Check sheet for the modelled part. Datum: model origin and axes. Units: mm. Face numbers are marked on the shaded views. A direction names the side the tool comes from. Round coordinates to 2 decimals unless told otherwise and drop trailing zeros. Write item = value, one per line.
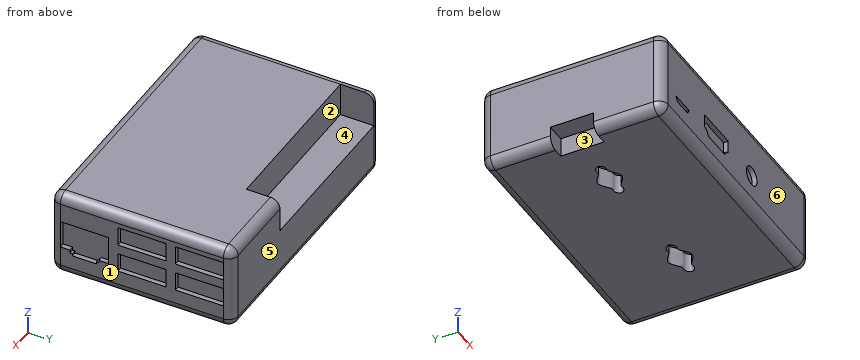
from build123d import *

# Parameters (mm, degrees)
F0_W     = 6.35
F0_H     = 7.14375
F1_DEPTH = 28.575
F2_DEPTH = 6.35
F4_W     = 15.875
F4_H     = 6.35
F5_DEPTH = 1.5875
F3_R     = 3.175
F6_DEPTH = 1.5875
F7_W     = 57.15
F7_H     = 11.1125
F8_DEPTH = 11.1125
F9_R     = 3.17499


# Not quite as in the source:
# - a fillet or chamfer is up to 0.001 mm smaller than in the source, because OpenCascade refuses the exact size


with BuildPart() as f1:
    # F0 (on Top) → F1 (new body)
    with BuildSketch(Plane.XY):
        Polygon((44.45, -30.1625), (44.45, 30.1625), (-44.45, 30.1625), (-44.45, 7.14375), (-38.1, 7.14375), (-38.1, 0), (-38.1, -7.14375), (-44.45, -7.14375), (-44.45, -30.1625), align=None)
        with BuildLine():
            add(Edge.make_bspline(
                [(-14.2875, 0), (-14.2875, 0.7324493897), (-15.9479784808, 2.0808128457), (-17.5976715514, 0.8021829538), (-21.43125, 5.9657530394), (-25.2648284486, 0.8021829538), (-26.9145215192, 2.0808128457), (-29.4769945213, 0), (-26.9145215192, -2.0808128457), (-25.2648284486, -0.8021829538), (-21.43125, -5.9657530394), (-17.5976715514, -0.8021829538), (-15.9479784808, -2.0808128457), (-14.2875, -0.7324493897), (-14.2875, 0)],
                knots=[0, 0, 0, 0, 0.0762961044, 0.1404532251, 0.25, 0.3595467749, 0.4237038956, 0.5, 0.5762961044, 0.6404532251, 0.75, 0.8595467749, 0.9237038956, 1, 1, 1, 1], degree=3))
        make_face(mode=Mode.SUBTRACT)
        with BuildLine():
            add(Edge.make_bspline(
                [(14.2875, 0), (14.2875, 0.7324493897), (15.9479784808, 2.0808128457), (17.5976715514, 0.8021829538), (21.43125, 5.9657530394), (25.2648284486, 0.8021829538), (26.9145215192, 2.0808128457), (29.4769945213, 0), (26.9145215192, -2.0808128457), (25.2648284486, -0.8021829538), (21.43125, -5.9657530394), (17.5976715514, -0.8021829538), (15.9479784808, -2.0808128457), (14.2875, -0.7324493897), (14.2875, 0)],
                knots=[0, 0, 0, 0, 0.0762961044, 0.1404532251, 0.25, 0.3595467749, 0.4237038956, 0.5, 0.5762961044, 0.6404532251, 0.75, 0.8595467749, 0.9237038956, 1, 1, 1, 1], degree=3))
        make_face(mode=Mode.SUBTRACT)
        with Locations((-41.275, 3.571875)):
            Rectangle(F0_W, F0_H)
        with Locations((-41.275, -3.571875)):
            Rectangle(F0_W, F0_H)
        with BuildLine():
            add(Edge.make_bspline(
                [(-14.2875, 0), (-14.2875, 0.7324493897), (-15.9479784808, 2.0808128457), (-17.5976715514, 0.8021829538), (-21.43125, 5.9657530394), (-25.2648284486, 0.8021829538), (-26.9145215192, 2.0808128457), (-29.4769945213, 0), (-26.9145215192, -2.0808128457), (-25.2648284486, -0.8021829538), (-21.43125, -5.9657530394), (-17.5976715514, -0.8021829538), (-15.9479784808, -2.0808128457), (-14.2875, -0.7324493897), (-14.2875, 0)],
                knots=[0, 0, 0, 0, 0.0762961044, 0.1404532251, 0.25, 0.3595467749, 0.4237038956, 0.5, 0.5762961044, 0.6404532251, 0.75, 0.8595467749, 0.9237038956, 1, 1, 1, 1], degree=3))
        make_face()
        with BuildLine():
            add(Edge.make_bspline(
                [(14.2875, 0), (14.2875, 0.7324493897), (15.9479784808, 2.0808128457), (17.5976715514, 0.8021829538), (21.43125, 5.9657530394), (25.2648284486, 0.8021829538), (26.9145215192, 2.0808128457), (29.4769945213, 0), (26.9145215192, -2.0808128457), (25.2648284486, -0.8021829538), (21.43125, -5.9657530394), (17.5976715514, -0.8021829538), (15.9479784808, -2.0808128457), (14.2875, -0.7324493897), (14.2875, 0)],
                knots=[0, 0, 0, 0, 0.0762961044, 0.1404532251, 0.25, 0.3595467749, 0.4237038956, 0.5, 0.5762961044, 0.6404532251, 0.75, 0.8595467749, 0.9237038956, 1, 1, 1, 1], degree=3))
        make_face()
    extrude(amount=F1_DEPTH)

    # F0 (on Top) → F2 (cut)
    with BuildSketch(Plane.XY):
        with Locations((-41.275, 3.571875)):
            Rectangle(F0_W, F0_H)
        with Locations((-41.275, -3.571875)):
            Rectangle(F0_W, F0_H)
        with BuildLine():
            add(Edge.make_bspline(
                [(-14.2875, 0), (-14.2875, 0.7324493897), (-15.9479784808, 2.0808128457), (-17.5976715514, 0.8021829538), (-21.43125, 5.9657530394), (-25.2648284486, 0.8021829538), (-26.9145215192, 2.0808128457), (-29.4769945213, 0), (-26.9145215192, -2.0808128457), (-25.2648284486, -0.8021829538), (-21.43125, -5.9657530394), (-17.5976715514, -0.8021829538), (-15.9479784808, -2.0808128457), (-14.2875, -0.7324493897), (-14.2875, 0)],
                knots=[0, 0, 0, 0, 0.0762961044, 0.1404532251, 0.25, 0.3595467749, 0.4237038956, 0.5, 0.5762961044, 0.6404532251, 0.75, 0.8595467749, 0.9237038956, 1, 1, 1, 1], degree=3))
        make_face()
        with BuildLine():
            add(Edge.make_bspline(
                [(14.2875, 0), (14.2875, 0.7324493897), (15.9479784808, 2.0808128457), (17.5976715514, 0.8021829538), (21.43125, 5.9657530394), (25.2648284486, 0.8021829538), (26.9145215192, 2.0808128457), (29.4769945213, 0), (26.9145215192, -2.0808128457), (25.2648284486, -0.8021829538), (21.43125, -5.9657530394), (17.5976715514, -0.8021829538), (15.9479784808, -2.0808128457), (14.2875, -0.7324493897), (14.2875, 0)],
                knots=[0, 0, 0, 0, 0.0762961044, 0.1404532251, 0.25, 0.3595467749, 0.4237038956, 0.5, 0.5762961044, 0.6404532251, 0.75, 0.8595467749, 0.9237038956, 1, 1, 1, 1], degree=3))
        make_face()
    extrude(amount=F2_DEPTH, mode=Mode.SUBTRACT)

    # F4 (on face) → F5 (cut)
    with BuildSketch(Plane.YZ.offset(44.45)):
        with Locations((19.05, 11.1125)):
            Rectangle(F4_W, F4_H)
        with Locations((19.05, 20.6375)):
            Rectangle(F4_W, F4_H)
        with Locations((0, 11.1125)):
            Rectangle(F4_W, F4_H)
        with Locations((0, 20.6375)):
            Rectangle(F4_W, F4_H)
        Polygon((-11.1125, 19.05), (-26.9875, 19.05), (-26.9875, 9.7991283983), (-23.8125, 9.7991283983), (-23.8125, 8.73125), (-23.01875, 8.73125), (-23.01875, 7.9375), (-15.08125, 7.9375), (-15.08125, 8.73125), (-14.2875, 8.73125), (-14.2875, 9.4989752397), (-11.1125, 9.4989752397), align=None)
    extrude(amount=-F5_DEPTH, mode=Mode.SUBTRACT)

    # F3 (on face) → F6 (cut)
    with BuildSketch(Plane.XZ.offset(30.1625)):
        Polygon((-28.575, 9.525), (-36.5125, 9.525), (-35.71875, 7.9375), (-29.36875, 7.9375), align=None)
        with BuildLine():
            Line((-4.7625, 14.2875), (-19.05, 14.2875))
            Line((-19.05, 14.2875), (-19.05, 9.8425))
            ThreePointArc((-19.05, 9.8425), (-17.7029615818, 9.2845384182), (-17.145, 7.9375))
            Line((-17.145, 7.9375), (-6.6675, 7.9375))
            ThreePointArc((-6.6675, 7.9375), (-6.1095384182, 9.2845384182), (-4.7625, 9.8425))
            Line((-4.7625, 9.8425), (-4.7625, 14.2875))
        make_face()
        with Locations((9.525, 11.1125)):
            Circle(F3_R)
    extrude(amount=-F6_DEPTH, mode=Mode.SUBTRACT)

    # F7 (on face) → F8 (cut)
    with BuildSketch(Plane.XY.offset(28.575)):
        with Locations((-12.7, 24.60625)):
            Rectangle(F7_W, F7_H)
    extrude(amount=-F8_DEPTH, mode=Mode.SUBTRACT)

    # F9 (radius 3.175 in the source; OpenCascade refuses exactly that, so slightly less here)
    f9_edges = [f1.edges().sort_by_distance(p)[0] for p in [
        (0, -30.1625, 28.575),
        (-44.45, 0, 28.575),
        (44.45, 0, 28.575),
        (44.45, -30.1625, 14.2875),
        (0, -30.1625, 0),
        (44.45, 0, 0),
        (44.45, 30.1625, 14.2875),
        (-42.8625, 30.1625, 28.575),
        (30.1625, 30.1625, 28.575),
        (0, 30.1625, 0),
        (-44.45, 30.1625, 14.2875),
        (-44.45, 18.653125, 0),
        (-44.45, -18.653125, 0),
        (-44.45, -30.1625, 14.2875),
    ]]
    fillet(f9_edges, radius=F9_R)


solid = f1.part
(1) Access from +Z, -Z, +X, -X, +Y, -Y to the whole of each face (thin tool, end or side, straight path). Record for the marked faces 1 and 2.
Worked answers:
face_1 = +Z, -Z, +X, +Y, -Y
face_2 = +Z, +Y
(2) Go/stop test with flat-tipped pins: P1, Ø12, axis at x = -11, y = 25.5, coming from the +Z side; P2, Ø0.5, axis at x = 43.5, z = 12.5, coming from the -Y side; P3, Ø0.8, axis at x = 43.5, z = 10, coming from the +Y side. Record where each tip stops, or that it passes through.
Worked answers:
P1 = 17.46
P2 = -29.47
P3 = 29.59
(3) Release check for a two-part mould opening along Y. For the marked faces 3, 4, 5 and 6 record: pulls with the +Y half, pulls with the -Y half, needs draft (parallel to the pull), parting line crosses it, or undercut.
Worked answers:
face_3 = undercut
face_4 = needs draft
face_5 = pulls with the +Y half
face_6 = pulls with the -Y half
(4) Material ranges on L1, parallel to X at y = -5, z = 5.75; L2, parallel to X at y = -4, z = 22.25; L3, parallel to Z at x = -18.5, y = 23, recorded low to high. Write a range as [from, to].
Worked answers:
L1 = [-38.1, 44.45]
L2 = [-44.45, 42.86]
L3 = [0, 17.46]
